The listing builds one solid part. Answer for the finished solid, in the listing's coordinates (mm). A direction names the side the tool comes from. Coordinates: 2 decimals unless noted, no trailing zeros. Write each loop counter-clockwise with the first axis right and the second up, starting at its lowest first coordinate (ties: lowest second). Pieces come first, ordered by that corner, then holes.
```python
from build123d import *

# Parameters (mm, degrees)
SKETCH_1_W               = 240
SKETCH_1_H               = 170
SKETCH_1_R               = 2.15
EXTRUDE_1_DEPTH          = 80
SKETCH_2_W               = 230
SKETCH_2_H               = 160
CUT_EXTRUDE_1_DEPTH      = 75
CUT_EXTRUDE_3_DEPTH      = 220.146070008
CUT_EXTRUDE_3_DEPTH_BACK = 220.146070008
FILLET_1_R               = 5
SKETCH_12_W              = 244.6
SKETCH_12_H              = 174.6
CUT_EXTRUDE_5_DEPTH      = 15


with BuildPart() as part:
    # 草图1 → 凸台-拉伸1 (new body)
    with BuildSketch(Plane(origin=(0, 0, 0), x_dir=(1, 0, 0), z_dir=(0, 1, 0))):
        Rectangle(SKETCH_1_W, SKETCH_1_H)
        with Locations(Location((-105.882352941, 75, 0), (0, 0, 270))):
            Circle(SKETCH_1_R, mode=Mode.SUBTRACT)
        with Locations(Location((105.882352941, 75, 0), (0, 0, 270))):
            Circle(SKETCH_1_R, mode=Mode.SUBTRACT)
        with Locations(Location((105.882352941, -75, 0), (0, 0, 270))):
            Circle(SKETCH_1_R, mode=Mode.SUBTRACT)
        with Locations(Location((-105.882352941, -75, 0), (0, 0, 270))):
            Circle(SKETCH_1_R, mode=Mode.SUBTRACT)
    extrude(amount=EXTRUDE_1_DEPTH)

    # 草图2 → 切除-拉伸1 (cut)
    with BuildSketch(Plane(origin=(0, 80, 0), x_dir=(1, 0, 0), z_dir=(0, 1, 0))):
        Rectangle(SKETCH_2_W, SKETCH_2_H)
    extrude(amount=-CUT_EXTRUDE_1_DEPTH, mode=Mode.SUBTRACT)

    # 草图9 → 切除-拉伸3 (cut, two sides: drawn at the far end of the back side and taken through both)
    with BuildSketch(Plane.XY.offset(-80).offset(-CUT_EXTRUDE_3_DEPTH_BACK)):
        with BuildLine():
            Line((-115, 26), (-115, 34))
            ThreePointArc((-115, 34), (-107.5, 41.5), (-100, 34))
            Line((-100, 34), (-100, 26))
            ThreePointArc((-100, 26), (-107.5, 18.5), (-115, 26))
        make_face()
        with BuildLine():
            Line((-7.5, 26), (-7.5, 34))
            ThreePointArc((-7.5, 34), (0, 41.5), (7.5, 34))
            Line((7.5, 34), (7.5, 26))
            ThreePointArc((7.5, 26), (0, 18.5), (-7.5, 26))
        make_face()
    extrude(amount=CUT_EXTRUDE_3_DEPTH + CUT_EXTRUDE_3_DEPTH_BACK, mode=Mode.SUBTRACT)

    # 圆角1
    fillet_1_edges = [part.edges().sort_by_distance(p)[0] for p in [
        (-115, 15.5, 80),
        (-115, 15.5, -80),
        (115, 42.5, -80),
        (115, 42.5, 80),
        (-115, 57, -80),
        (120, 40, 85),
        (-120, 40, 85),
        (-120, 40, -85),
        (120, 40, -85),
    ]]
    fillet(fillet_1_edges, radius=FILLET_1_R - 0.0001)  # a hair under: the kernel refuses the full size

    # 草图12 → 切除-拉伸5 (cut)
    # profile 1 of 2: a face of its own
    with BuildSketch(Plane(origin=(0, 80, 0), x_dir=(1, 0, 0), z_dir=(0, 1, 0))):
        Rectangle(SKETCH_12_W, SKETCH_12_H)
        with BuildLine():
            Line((115, 85), (-115, 85))
            ThreePointArc((-115, 85), (-118.535533906, 83.535533906), (-120, 80))
            Line((-120, 80), (-120, -80))
            ThreePointArc((-120, -80), (-118.535533906, -83.535533906), (-115, -85))
            Line((-115, -85), (115, -85))
            ThreePointArc((115, -85), (118.535533906, -83.535533906), (120, -80))
            Line((120, -80), (120, 80))
            ThreePointArc((120, 80), (118.535533906, 83.535533906), (115, 85))
        make_face(mode=Mode.SUBTRACT)
    # profile 2 of 2: a face of its own
    with BuildSketch(Plane(origin=(0, 80, 0), x_dir=(1, 0, 0), z_dir=(0, 1, 0))):
        with BuildLine():
            ThreePointArc((120, 80), (118.535533906, 83.535533906), (115, 85))
            Line((115, 85), (-115, 85))
            ThreePointArc((-115, 85), (-118.535533906, 83.535533906), (-120, 80))
            Line((-120, 80), (-120, -80))
            ThreePointArc((-120, -80), (-118.535533906, -83.535533906), (-115, -85))
            Line((-115, -85), (115, -85))
            ThreePointArc((115, -85), (118.535533906, -83.535533906), (120, -80))
            Line((120, -80), (120, 80))
        make_face()
        with BuildLine():
            ThreePointArc((-112.3, 82.3), (-115.835533906, 80.835533906), (-117.3, 77.3))
            Line((-117.3, 77.3), (-117.3, -77.3))
            ThreePointArc((-117.3, -77.3), (-115.835533906, -80.835533906), (-112.3, -82.3))
            Line((-112.3, -82.3), (112.3, -82.3))
            ThreePointArc((112.3, -82.3), (115.835533906, -80.835533906), (117.3, -77.3))
            Line((117.3, -77.3), (117.3, 77.3))
            ThreePointArc((117.3, 77.3), (115.835533906, 80.835533906), (112.3, 82.3))
            Line((112.3, 82.3), (-112.3, 82.3))
        make_face(mode=Mode.SUBTRACT)
    extrude(amount=-CUT_EXTRUDE_5_DEPTH, mode=Mode.SUBTRACT)


solid = part.part
```
(1) Which of the six approach directions +Z, -Z, +X, -X, +Y, -Y give full straight-line access (tool end or side, diameter ignored) to faces 4 (the flat face through (7.5, 30, 82)), 5 (the cylindrical face through (-115.87, 72.6, 80.8)), 6 (the cylindrical face through (115.8, 72.6, 80.87)), 7 (the flat face through (2, 73, -82.3)), 8 (the cylindrical face through (115.87, 72.6, -80.8))?
(2) Section A-A, the plane x = 0 is taken. Write down the section's boundary in (y, z).
(3) Section C-C, the plane z = -25 is taken. Write down the section's boundary in (x, y).
(4) Each of these flat-tipped pins is pushed along its axis until it touches: pin 1 (1 mm diameter, centred on x = 74, z = -32, fed in from +Y); pin 2 (4 mm diameter, centred on y = 28, z = 82.5, fed in from -X); pin 3 (5.5 mm diameter, centred on y = 31, z = -83.5, fed in from -X). Where does it stop, or does it pass through?
(5) Section B-B, the plane y = 8 is taken. Write down the section's boundary in (x, z), plus the area to 3 significant figures.
(6) For a pull along Z with two mould halves and no side action, classify faces 1 (the cylindrical face through (113, 42, 79)), 2 (the flat face through (-7.5, 30, -83)), 3 (the flat face through (-2, 18, 85)) as pulls with the +Z half, pulls with the -Z half, needs draft (parallel to the pull), parting line crosses it, or undercut.
(7) Find the intervals of material crossed by probe 1 along X at (y, z) = (1.9, -75); probe 2 along Z at (x, y) = (-45.5, 69.5); probe 3 along X at (y, z) = (22.5, -15), in increasing order.
Solution:
1. face 4: +Z, -Z
1. face 5: +Z, -X, +Y
1. face 6: +Z, +X, +Y
1. face 7: -Z, +X, -X, +Y
1. face 8: -Z, +X, +Y
2. outline: (0, -85) - (18.5, -85) - (18.5, -80) - (5, -80) - (5, 80) - (18.5, 80) - (18.5, 85) - (0, 85) - close; (41.5, -85) - (65, -85) - (65, -82.3) - (80, -82.3) - (80, -80) - (41.5, -80) - close; (41.5, 80) - (80, 80) - (80, 82.3) - (65, 82.3) - (65, 85) - (41.5, 85) - close
3. outline: (-120, 0) - (120, 0) - (120, 65) - (117.3, 65) - (117.3, 80) - (115, 80) - (115, 5) - (-115, 5) - (-115, 80) - (-117.3, 80) - (-117.3, 65) - (-120, 65) - close
4. pin 1: stops at y = 5
4. pin 2: stops at x = -119.97
4. pin 3: stops at x = -119.94
5. outline: (-120, -80) arc R5 ccw to (-115, -85) - (115, -85) arc R5 ccw to (120, -80) - (120, 80) arc R5 ccw to (115, 85) - (-115, 85) arc R5 ccw to (-120, 80) - close; hole (-115, -75) arc R5 ccw to (-110, -80) - (110, -80) arc R5 ccw to (115, -75) - (115, 75) arc R5 ccw to (110, 80) - (-110, 80) arc R5 ccw to (-115, 75) - close
5. area: 4,000 mm2
6. face 1: undercut
6. face 2: needs draft
6. face 3: pulls with the +Z half
7. probe 1: x = -120 to -108.03, -103.73 to 103.73, 108.03 to 120
7. probe 2: z = -82.3 to -80, 80 to 82.3
7. probe 3: x = -120 to -115, 115 to 120
